For this review, take the finished solid that the model builds, in its own axes (mm). Round coordinates to 2 decimals unless told otherwise and drop trailing zeros. Order: outer loops, then holes, each group sorted by start corner. A loop starts at its lowest first (then second) coordinate and runs counter-clockwise, first axis right, second up. Notation, with made-up numbers: M 89,-39.5 L 110,-39.5 A10 ccw 110,-28.5 Z; hole C -17,-9.75 d6. An arc over 180 degrees is marked long. Answer as a JSON object with one key per item and string values.
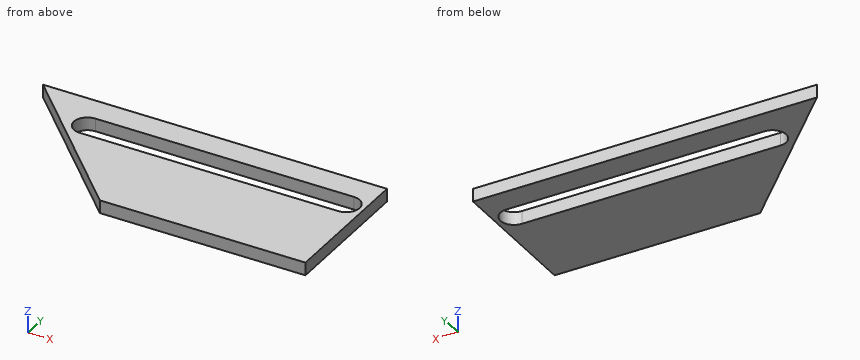
from build123d import *

# Parameters (mm, degrees)
BOSS_EXTRUDE1_DEPTH = 5


with BuildPart() as part:
    # Sketch1 → Boss-Extrude1 (new body)
    with BuildSketch(Plane.XY):
        Polygon((0, 0), (0, 54.5), (-133, 54.5), (-79.5, 0), align=None)
        with BuildLine():
            Line((-107, 44.5), (-7, 44.5))
            ThreePointArc((-7, 44.5), (-1.75, 39.25), (-7, 34))
            Line((-7, 34), (-107, 34))
            ThreePointArc((-107, 34), (-112.25, 39.25), (-107, 44.5))
        make_face(mode=Mode.SUBTRACT)
    extrude(amount=BOSS_EXTRUDE1_DEPTH)


solid = part.part
1) Add section C-C on y = 39.25. State the section outline as (x, z) points.
Geometry check:
{"outline": "M -118.03,0 L -112.25,0 L -112.25,5 L -118.03,5 Z; M -1.75,0 L 0,0 L 0,5 L -1.75,5 Z"}
2) Add section B-B on z = 0.85. State the section outline as (x, y) points.
Geometry check:
{"outline": "M -133,54.5 L -79.5,0 L 0,0 L 0,54.5 Z; hole M -107,34 L -7,34 A5.25 ccw -7,44.5 L -107,44.5 A5.25 ccw Z"}
3) Insertion check: P1, Ø1, axis at y = 43.5, z = 4, coming from the -X side; P2, Ø3, axis at x = -90, z = 2.5, coming from the -Y side. Each pin has a flat end and moves straight along its axis. Give the tip position at first contact, or say it passes through.
Geometry check:
{"P1": "stops at x = -122.69", "P2": "stops at y = 9.17"}
4) Add section D-D on y = 30.5. State the section outline as (x, z) points, and give its area (3 significant figures).
Geometry check:
{"outline": "M -109.44,0 L 0,0 L 0,5 L -109.44,5 Z", "area": "547 mm²"}
5) For L1, parallel to Y at x = -13.5, z = 4.2; L2, parallel to Y at x = -104, z = 2.65; L3, parallel to X at y = 39, z = 2.9, list the stretches that pass through material, from the lowest coordinate up.
Geometry check:
{"L1": "y = 0 to 34, 44.5 to 54.5", "L2": "y = 24.96 to 34, 44.5 to 54.5", "L3": "x = -117.78 to -112.24, -1.76 to 0"}
6) Add section A-A on x = -22. State the section outline as (y, z) points.
Geometry check:
{"outline": "M 0,0 L 34,0 L 34,5 L 0,5 Z; M 44.5,0 L 54.5,0 L 54.5,5 L 44.5,5 Z"}
